The listing builds one solid part. Answer for the finished solid, in the listing's coordinates (mm). Face numbers are marked on the shaded views. A direction names the side the tool comes from. Round coordinates to 2 decimals unless told otherwise and drop trailing zeros. Write each loop counter-clockwise with the first axis right and the second up, starting at its lowest first coordinate (ties: lowest second). Pieces come first, ordered by that corner, then holes. Notation, with made-up numbers: M 60.5,17 L 64.5,17 A25 cw 64.5,49 Z; hole C 83.25,22.25 d11. An arc over 180 degrees is marked long. Put each result on its own line as item: value. Start each with the question number.
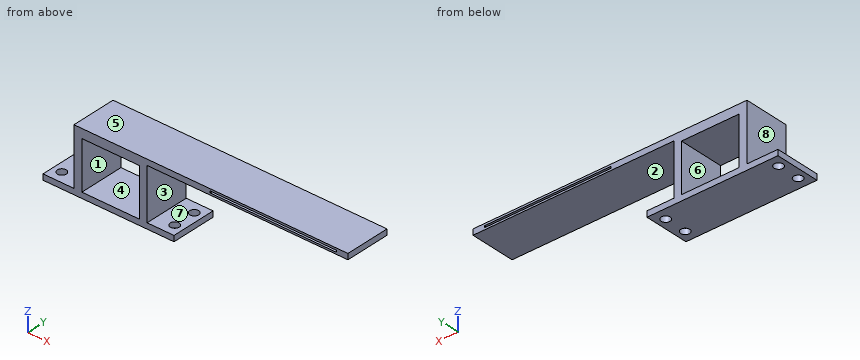
```python
from build123d import *

# Parameters (mm, degrees)
F0_W     = 58
F0_H     = 20
F0_R     = 2
F1_DEPTH = 2.54
F2_W     = 32.392131
F2_H     = 20
F3_DEPTH = 25.4
F4_W     = 20
F4_H     = 2.54
F5_DEPTH = 88.9
F6_W     = 56
F6_H     = 0.8
F7_DEPTH = 20.001
F8_W     = 25.481197
F8_H     = 21.373894
F9_DEPTH = 20.001


with BuildPart() as f1:
    # F0 (on Top) → F1 (new body)
    with BuildSketch(Plane.XY):
        Rectangle(F0_W, F0_H)
        with Locations((-25, -5)):
            Circle(F0_R, mode=Mode.SUBTRACT)
        with Locations((25, -5)):
            Circle(F0_R, mode=Mode.SUBTRACT)
        with Locations((-25, 5)):
            Circle(F0_R, mode=Mode.SUBTRACT)
        with Locations((25, 5)):
            Circle(F0_R, mode=Mode.SUBTRACT)
    extrude(amount=F1_DEPTH)

    # F2 (on face) → F3 (join)
    with BuildSketch(Plane.XY.offset(2.54)):
        with Locations((0.897951, 0)):
            Rectangle(F2_W, F2_H)
    extrude(amount=F3_DEPTH)

    # F4 (on face) → F5 (join)
    with BuildSketch(Plane.YZ.offset(17.094016)):
        with Locations((0, 26.67)):
            Rectangle(F4_W, F4_H)
    extrude(amount=F5_DEPTH)

    # F6 (on face) → F7 (cut, through all)
    with BuildSketch(Plane(origin=(0, 10, 0), x_dir=(-1, 0, 0), z_dir=(0, 1, 0))):
        with Locations((-72.994016, 26.651)):
            Rectangle(F6_W, F6_H)
    extrude(amount=-F7_DEPTH, mode=Mode.SUBTRACT)

    # F8 (on face) → F9 (cut, through all)
    with BuildSketch(Plane.XZ.offset(10)):
        with Locations((0.961546, 13.226947)):
            Rectangle(F8_W, F8_H)
    extrude(amount=-F9_DEPTH, mode=Mode.SUBTRACT)


solid = f1.part
```
Item 1: Which of the six approach directions +Z, -Z, +X, -X, +Y, -Y give full straight-line access (tool end or side, diameter ignored) to the marked faces 5, 6, 7 and 8?
Item 2: Section D-D (x = 54.5) is taken. Give the vertices of the cut face in (y, z).
Item 3: Flat-ended cylindrical pins translate along their axes: pin 1 (0.9 mm diameter, centred on y = -5, z = 27, fed in from -X); pin 2 (6.5 mm diameter, centred on x = -25, y = 5, fed in from +Z); pin 3 (1.5 mm diameter, centred on x = 46.5, y = 4, fed in from -Z); pin 4 (3 mm diameter, centred on x = -25, y = -5, fed in from -Z). Find the tip coordinate at first contact, or state that the pin passes through.
Item 4: Section A-A (x = 25) is taken. Give the vertices of the cut face in (y, z).
Item 5: Section B-B (y = -5) is taken. Give the vertices of the cut face in (x, z).
Item 6: Determine the mould class of the marked faces 1, 2, 3 and 4 for opening direction X: released by +X, released by -X, zero draft, split by the parting line, or undercut.
Item 7: Consider line 1 along Y through (x, z) = (-25, 0.85); line 2 along X through (y, z) = (-1.5, 15.5); line 3 along Y through (x, z) = (24, 2.5). Determine where each line is inside the solid, lowest interval first. Write a range as [from, to].
Item 8: Section C-C (z = 5.75) is taken. Give the vertices of the cut face in (x, y).
Output values:
1. face 5: +Z, +X, -X, +Y, -Y
1. face 6: +Y, -Y
1. face 7: +X, +Y, -Y
1. face 8: +Z, -X, +Y, -Y
2. outline: M -10,25.4 L 10,25.4 L 10,26.25 L -10,26.25 Z; M -10,27.05 L 10,27.05 L 10,27.94 L -10,27.94 Z
3. pin 1: stops at x = -15.3
3. pin 2: stops at z = 2.54
3. pin 3: stops at z = 25.4
3. pin 4: passes through
4. outline: M -10,0 L -7,0 L -7,2.54 L -10,2.54 Z; M -10,25.4 L 10,25.4 L 10,27.94 L -10,27.94 Z; M -3,0 L 3,0 L 3,2.54 L -3,2.54 Z; M 7,0 L 10,0 L 10,2.54 L 7,2.54 Z
5. outline: M -29,0 L -27,0 L -27,2.54 L -29,2.54 Z; M -23,0 L 23,0 L 23,2.54 L 17.09,2.54 L 17.09,25.4 L 105.99,25.4 L 105.99,27.94 L -15.3,27.94 L -15.3,2.54 L -23,2.54 Z; M 27,0 L 29,0 L 29,2.54 L 27,2.54 Z; hole M -11.78,2.54 L 13.7,2.54 L 13.7,23.91 L -11.78,23.91 Z; hole M 44.99,26.25 L 100.99,26.25 L 100.99,27.05 L 44.99,27.05 Z
6. face 1: undercut
6. face 2: zero draft
6. face 3: released by +X
6. face 4: undercut
7. line 1: y = [-10, -7], [-3, 3], [7, 10]
7. line 2: x = [-15.3, -11.78], [13.7, 17.09]
7. line 3: y = [-10, -6.73], [-3.27, 3.27], [6.73, 10]
8. outline: M -15.3,-10 L -11.78,-10 L -11.78,10 L -15.3,10 Z; M 13.7,-10 L 17.09,-10 L 17.09,10 L 13.7,10 Z
